from build123d import *

# Parameters (mm, degrees)
SKETCH_1_R      = 0.6
EXTRUDE_1_DEPTH = 2
EXTRUDE_2_DEPTH = 7


with BuildPart() as part:
    # Эскиз1 → Бобышка-Вытянуть1 (new body)
    with BuildSketch(Plane.XY):
        with BuildLine():
            Line((9.649784207, -2.239485083), (4.657979857, -4.056353282))
            ThreePointArc((4.657979857, -4.056353282), (4.180847956, -4.422469466), (4, -4.996045902))
            Line((4, -4.996045902), (4, -13.640598923))
            Line((4, -13.640598923), (0, -15.95))
            Line((0, -15.95), (0, -18.95))
            Line((0, -18.95), (21.7, -18.95))
            Line((21.7, -18.95), (21.7, 18.95))
            Line((21.7, 18.95), (0, 18.95))
            Line((0, 18.95), (0, 15.95))
            Line((0, 15.95), (4, 13.640598923))
            Line((4, 13.640598923), (4, 4.996045902))
            ThreePointArc((4, 4.996045902), (4.180847956, 4.422469466), (4.657979857, 4.056353282))
            Line((4.657979857, 4.056353282), (9.649784207, 2.239485083))
            ThreePointArc((9.649784207, 2.239485083), (10.126916108, 1.873368898), (10.307764064, 1.299792462))
            Line((10.307764064, 1.299792462), (10.307764064, -1.299792462))
            ThreePointArc((10.307764064, -1.299792462), (10.126916108, -1.873368898), (9.649784207, -2.239485083))
        make_face()
        with Locations((2.4, -16.95)):
            Circle(SKETCH_1_R, mode=Mode.SUBTRACT)
        with Locations((2.4, 16.95)):
            Circle(SKETCH_1_R, mode=Mode.SUBTRACT)
        with Locations((19.3, -16.95)):
            Circle(SKETCH_1_R, mode=Mode.SUBTRACT)
        with Locations((19.3, 16.95)):
            Circle(SKETCH_1_R, mode=Mode.SUBTRACT)
        with BuildLine():
            Line((4.8, -18.15), (15.9, -18.15))
            Line((15.9, -18.15), (20.9, -13.15))
            Line((20.9, -13.15), (20.9, 13.15))
            Line((20.9, 13.15), (15.9, 18.15))
            Line((15.9, 18.15), (4.8, 18.15))
            Line((4.8, 18.15), (4.8, 14.102479139))
            Line((4.8, 14.102479139), (4.8, 4.996045902))
            ThreePointArc((4.8, 4.996045902), (4.836169591, 4.881330615), (4.931595971, 4.808107378))
            Line((4.931595971, 4.808107378), (9.923400322, 2.991239179))
            ThreePointArc((9.923400322, 2.991239179), (10.782237744, 2.332230047), (11.107764064, 1.299792462))
            Line((11.107764064, 1.299792462), (11.107764064, -1.299792462))
            ThreePointArc((11.107764064, -1.299792462), (10.782237744, -2.332230047), (9.923400322, -2.991239179))
            Line((9.923400322, -2.991239179), (4.931595971, -4.808107378))
            ThreePointArc((4.931595971, -4.808107378), (4.836169591, -4.881330615), (4.8, -4.996045902))
            Line((4.8, -4.996045902), (4.8, -14.102479139))
            Line((4.8, -14.102479139), (4.8, -18.15))
        make_face(mode=Mode.SUBTRACT)
    extrude(amount=EXTRUDE_1_DEPTH)

    # Эскиз3 → Бобышка-Вытянуть2 (add)
    with BuildSketch(Plane.XY.offset(2)):
        with BuildLine():
            Line((9.649784207, -2.239485083), (4.657979857, -4.056353282))
            ThreePointArc((4.657979857, -4.056353282), (4.180847956, -4.422469466), (4, -4.996045902))
            Line((4, -4.996045902), (4, -13.640598923))
            Line((4, -13.640598923), (0, -15.95))
            Line((0, -15.95), (0, -18.95))
            Line((0, -18.95), (21.7, -18.95))
            Line((21.7, -18.95), (21.7, 18.95))
            Line((21.7, 18.95), (0, 18.95))
            Line((0, 18.95), (0, 15.95))
            Line((0, 15.95), (4, 13.640598923))
            Line((4, 13.640598923), (4, 4.996045902))
            ThreePointArc((4, 4.996045902), (4.180847956, 4.422469466), (4.657979857, 4.056353282))
            Line((4.657979857, 4.056353282), (9.649784207, 2.239485083))
            ThreePointArc((9.649784207, 2.239485083), (10.126916108, 1.873368898), (10.307764064, 1.299792462))
            Line((10.307764064, 1.299792462), (10.307764064, -1.299792462))
            ThreePointArc((10.307764064, -1.299792462), (10.126916108, -1.873368898), (9.649784207, -2.239485083))
        make_face()
        with BuildLine():
            Line((0.8, -18.15), (20.9, -18.15))
            Line((20.9, -18.15), (20.9, 18.15))
            Line((20.9, 18.15), (0.8, 18.15))
            Line((0.8, 18.15), (0.8, 16.411880215))
            Line((0.8, 16.411880215), (4.8, 14.102479139))
            Line((4.8, 14.102479139), (4.8, 4.996045902))
            ThreePointArc((4.8, 4.996045902), (4.836169591, 4.881330615), (4.931595971, 4.808107378))
            Line((4.931595971, 4.808107378), (9.923400322, 2.991239179))
            ThreePointArc((9.923400322, 2.991239179), (10.782237744, 2.332230047), (11.107764064, 1.299792462))
            Line((11.107764064, 1.299792462), (11.107764064, -1.299792462))
            ThreePointArc((11.107764064, -1.299792462), (10.782237744, -2.332230047), (9.923400322, -2.991239179))
            Line((9.923400322, -2.991239179), (4.931595971, -4.808107378))
            ThreePointArc((4.931595971, -4.808107378), (4.836169591, -4.881330615), (4.8, -4.996045902))
            Line((4.8, -4.996045902), (4.8, -14.102479139))
            Line((4.8, -14.102479139), (0.8, -16.411880215))
            Line((0.8, -16.411880215), (0.8, -18.15))
        make_face(mode=Mode.SUBTRACT)
    extrude(amount=EXTRUDE_2_DEPTH)


solid = part.part
The listing builds one solid part. Answer for the finished solid, in the listing's coordinates (mm). A direction names the side the tool comes from. Coordinates: 2 decimals unless noted, no trailing zeros. Write each loop counter-clockwise with the first axis right and the second up, starting at its lowest first coordinate (ties: lowest second). Pieces come first, ordered by that corner, then holes. Notation, with made-up numbers: M 11.5,53 L 37.5,53 A14 ccw 37.5,60 Z; hole C 73,51 d10. An arc over 180 degrees is marked long. Write each question's results on one line, items separated by ' | '.
Item 1: Which of the six approach directions +Z, -Z, +X, -X, +Y, -Y give full straight-line access (tool end or side, diameter ignored) to faces 4 (the face through (10.8, -1.3, 0)), 5 (the face through (10.308, 0, 4)), 6 (the face through (10.8, 0.1, 9)), 7 (the face through (18.43, 15.62, 0.99)), 8 (the face through (11, 18.15, 4))?
Answer below:
face 4: -Z, +X, -X, +Y, -Y | face 5: +Z, -Z, -X | face 6: +Z, +X, -X, +Y, -Y | face 7: +Z, -Z | face 8: +Z
Item 2: The part is cut by section A-A on y = -6.5. Determine the outline of the cut face in (x, z).
Answer below:
outline: M 4,0 L 4.8,0 L 4.8,9 L 4,9 Z; M 20.9,0 L 21.7,0 L 21.7,9 L 20.9,9 Z
Item 3: Consider probe 1 along Y at (x, z) = (19.5, 4); probe 2 along X at (y, z) = (-6.5, 4); probe 3 along Y at (x, z) = (19.3, 1.15). Determine where each line is inside the solid, lowest interval first. Write a range as [from, to].
Answer below:
probe 1: [-18.95, -18.15], [18.15, 18.95] | probe 2: [4, 4.8], [20.9, 21.7] | probe 3: [-18.95, -17.55], [-16.35, -14.75], [14.75, 16.35], [17.55, 18.95]
Item 4: Given P1, Ø0.8, axis at y = -0.5, z = 3, coming from the -X side; P2, Ø4.5, axis at y = 7.5, z = 3.5, coming from the -X side; P3, Ø2.5, axis at x = 18, y = 16, coming from the +Z side, each flat-ended and moving along its own axis, determine where each tip first touches the part or whether it passes through.
Answer below:
P1: x = 10.31 | P2: x = 4 | P3: z = 2
Item 5: The part is cut by section C-C on y = 16.95. Determine the outline of the cut face in (x, z), and give its area (3 significant figures).
Answer below:
outline: M 0,0 L 1.8,0 L 1.8,2 L 0.8,2 L 0.8,9 L 0,9 Z; M 3,0 L 4.8,0 L 4.8,2 L 3,2 Z; M 17.1,0 L 18.7,0 L 18.7,2 L 17.1,2 Z; M 19.9,0 L 21.7,0 L 21.7,9 L 20.9,9 L 20.9,2 L 19.9,2 Z | area: 25.2 mm2
Item 6: For a pull along Y with two mould halves and no side action, classify faces 1 (the face through (0, 17, 4)), 2 (the face through (11, -18.95, 4)), 3 (the face through (7.189, -3.135, 4.437)) as released by +Y, released by -Y, zero draft, split by the parting line, or undercut.
Answer below:
face 1: zero draft | face 2: released by -Y | face 3: undercut
Item 7: The part is cut by section D-D on x = 19.3. Determine the outline of the cut face in (y, z).
Answer below:
outline: M -18.95,0 L -17.55,0 L -17.55,2 L -18.15,2 L -18.15,9 L -18.95,9 Z; M -16.35,0 L -14.75,0 L -14.75,2 L -16.35,2 Z; M 14.75,0 L 16.35,0 L 16.35,2 L 14.75,2 Z; M 17.55,0 L 18.95,0 L 18.95,9 L 18.15,9 L 18.15,2 L 17.55,2 Z
